```python
from build123d import *

# Parameters (mm, degrees)
F0_W     = 30
F0_H     = 5
F1_DEPTH = 34
F0_H_2   = 12
F0_R     = 1.75
F2_DEPTH = 5
F3_W     = 30
F3_H     = 5
F3_H_2   = 66
F4_DEPTH = 5
F5_R     = 4


with BuildPart() as f1:
    # F0 (on Top) → F1 (new body)
    with BuildSketch(Plane.XY):
        with Locations((15, 68.5)):
            Rectangle(F0_W, F0_H)
    extrude(amount=F1_DEPTH)

    # F0 (on Top) → F2 (join)
    with BuildSketch(Plane.XY):
        with Locations((15, 77)):
            Rectangle(F0_W, F0_H_2)
        with Locations((15, 77)):
            Circle(F0_R, mode=Mode.SUBTRACT)
    extrude(amount=F2_DEPTH)



with BuildPart() as f1b:
    # F0 (on Top) → F1, piece 2 (new body)
    with BuildSketch(Plane.XY):
        with Locations((15, 2.5)):
            Rectangle(F0_W, F0_H)
    extrude(amount=F1_DEPTH)

    # F0 (on Top) → F2, piece 2 (join)
    with BuildSketch(Plane.XY):
        with Locations((15, -6)):
            Rectangle(F0_W, F0_H_2)
        with Locations((15, -6)):
            Circle(F0_R, mode=Mode.SUBTRACT)
    extrude(amount=F2_DEPTH)


with BuildPart() as f1_1:
    add(f1.part)

    add(f1b.part)  # F4 merges F1b
    # F3 (on face) → F4 (join)
    with BuildSketch(Plane.XY.offset(34)):
        with Locations((15, 68.5)):
            Rectangle(F3_W, F3_H)
        with Locations((15, 33)):
            Rectangle(F3_W, F3_H_2)
    extrude(amount=F4_DEPTH)

    # F5
    f5_edges = [f1_1.edges().sort_by_distance(p)[0] for p in [
        (15, 0, 5),
        (15, 0, 39),
        (15, 71, 39),
        (15, 71, 5),
    ]]
    fillet(f5_edges, radius=F5_R)


solid = f1_1.part
```
Verification items for the finished model (mm, model axes). A direction names the side the tool comes from. Give positions to 0.01 mm unless a question says otherwise; leave off trailing zeros. Write each loop counter-clockwise with the first axis right and the second up, starting at its lowest first coordinate (ties: lowest second). Pieces come first, ordered by that corner, then holes. Notation, with made-up numbers: M -0.5,55 L 21.5,55 A21 ccw 21.5,59 Z; hole C 43.5,80 d9. An arc over 180 degrees is marked long. One line per question, with ' | ' between items.
1) Section check C-C on z = 22.5. Enter the section's corners in (x, y).
Result:
outline: M 0,0 L 30,0 L 30,5 L 0,5 Z; M 0,66 L 30,66 L 30,71 L 0,71 Z
2) Set-up check for faces 5 (the flat face through (15, 5, 17)), 6 (the flat face through (15, -12, 2)), 7 (the flat face through (15, 79, 5)), 8 (the flat face through (15, -8, 5)), 9 (the cylindrical face through (15.81, -7.55, 2.46)): record each of +Z, -Z, +X, -X, +Y, -Y from which the full face is reachable in a straight line by a thin tool's end or side.
Result:
face 5: -Z, +X, -X | face 6: +Z, -Z, +X, -X, -Y | face 7: +Z, +X, -X, +Y | face 8: +Z, +X, -X, -Y | face 9: +Z, -Z
3) Mould release check, pull along X, two halves, no side actions. Record for faces 1 (the flat face through (30, 35, 35)), 2 (the cylindrical face through (14.62, 75.29, 2.46)), 3 (the flat face through (15, 75, 0)), 4 (the flat face through (0, 36, 35)): released by +X, released by -X, zero draft, split by the parting line, or undercut.
Result:
face 1: released by +X | face 2: undercut | face 3: zero draft | face 4: released by -X
4) Section check B-B on x = 15. Enter the section's corners in (y, z), plus the area to 3 significant figures.
Result:
outline: M -12,0 L -7.75,0 L -7.75,5 L -12,5 Z; M -4.25,0 L 5,0 L 5,34 L 66,34 L 66,0 L 75.25,0 L 75.25,5 L 75,5 A4 cw 71,9 L 71,35 A4 ccw 67,39 L 4,39 A4 ccw 0,35 L 0,9 A4 cw -4,5 L -4.25,5 Z; M 78.75,0 L 83,0 L 83,5 L 78.75,5 Z | area: 780 mm2
5) Gauge pin test, flat ends, axial feed: pin 1 Ø4 at (x, y) = (11.5, -6.5) entering from +Z; pin 2 Ø2 at (x, z) = (21.5, 34.5) entering from +Y; pin 3 Ø8 at (y, z) = (10.5, 15) entering from +X; pin 4 Ø4 at (x, y) = (8.5, 70.5) entering from +Z. Record the tip position at first contact, or that the pin passes through.
Result:
pin 1: stops at z = 5 | pin 2: stops at y = 71 | pin 3: passes through | pin 4: stops at z = 38.71
6) Section check D-D on x = 25.5. Enter the section's corners in (y, z), plus the area to 3 significant figures.
Result:
outline: M -12,0 L 5,0 L 5,34 L 66,34 L 66,0 L 83,0 L 83,5 L 75,5 A4 cw 71,9 L 71,35 A4 ccw 67,39 L 4,39 A4 ccw 0,35 L 0,9 A4 cw -4,5 L -12,5 Z | area: 815 mm2
7) Thickness scan on line 1 along Y through (x, z) = (15, 3.55); line 2 along Y through (x, z) = (16, 19.5); line 3 along X through (y, z) = (77, 1). Record the ranges inside material, lowest first. Write a range as [from, to].
Result:
line 1: y = [-12, -7.75], [-4.25, 5], [66, 75.25], [78.75, 83] | line 2: y = [0, 5], [66, 71] | line 3: x = [0, 13.25], [16.75, 30]
8) Section check A-A on y = 77. Enter the section's corners in (x, z).
Result:
outline: M 0,0 L 13.25,0 L 13.25,5 L 0,5 Z; M 16.75,0 L 30,0 L 30,5 L 16.75,5 Z
